The model under review builds one solid part; all positions refer to its coordinate system, in mm. A direction names the side the tool comes from. Coordinates: 2 decimals unless noted, no trailing zeros. Loops run counter-clockwise (first coordinate to the right, second up) from the corner with the lowest first, then second, coordinate; pieces in that order, holes last. Notation, with made-up numbers: M -20,-1 L 3,-1 A34 cw 3,38 Z; hole C -2.75,71.25 d5. An arc over 180 degrees is marked long. Write item = value, one per line. Start each with the question number.
Q1. For faces 1 (the face through (288.161, -6.324, 4.032)), 2 (the face through (12.161, -6.324, 4.032)), 3 (the face through (275, -7, 3)), list the 3-axis set-ups (+Z, -Z, +X, -X, +Y, -Y) from which the entire face can be reached by the end or side of a thin tool; tool diameter is ignored.
Q2. We need section B-B on x = 42.5. Give the boundary of the cut face in (y, z), and give its area (3 significant figures).
Q3. Clearance check with flat-ended pins moving along their axes: pin 1 Ø1.7 at (x, y) = (160, -1) entering from +Z; pin 2 Ø5 at (x, y) = (248, -3) entering from +Z; pin 3 Ø3 at (x, y) = (266, -4.5) entering from +Z. State where each tip first meets the part, or that it passes through.
Q4. Mouldability with a two-part tool opening along X and no side actions: class faces 4 (the face through (312, 1, 0)), 5 (the face through (152, 0, -10)), 6 (the face through (0, 1, 0)), 7 (the face through (300.76, 4.17, 2.17)) as released by +X, released by -X, zero draft, split by the parting line, or undercut.
Q5. Wall thickness on probe 1 along X at (y, z) = (6.75, 1.75); probe 2 along X at (y, z) = (1.5, -4.5); probe 3 along Y at (x, z) = (187.5, 0): over which ranges is each line inside the solid? List them lowest first.
Q6. We need section A-A on x = 159. Give the boundary of the cut face in (y, z), and give its area (3 significant figures).
from build123d import *

# Parameters (mm, degrees)
CHAMFER1_SIZE      = 0.5
SKETCH3_W          = 1.5
SKETCH3_H          = 0.3
SKETCH9_W          = 60
SKETCH9_H          = 6
CUT_EXTRUDE2_DEPTH = 3.5
FILLET4_R          = 3
FILLET5_R          = 3
FILLET6_R          = 0.2


with BuildPart() as part:
    # Sketch1 → Revolve1 (revolve)
    with BuildSketch(Plane.XY, mode=Mode.PRIVATE) as revolve1_sk:
        Polygon((0, 0), (0, 7.5), (25, 7.5), (25, 9), (26, 10), (274, 10), (275, 9), (275, 7.5), (300, 7.5), (300, 5), (312, 5), (312, 0), align=None)
    revolve(revolve1_sk.sketch.rotate(Axis((0, 0, 0), (1, 0, 0)), 90), axis=Axis((0, 0, 0), (1, 0, 0)))

    # Chamfer1
    chamfer1_edges = [part.edges().sort_by_distance(p)[0] for p in [
        (300, 0, -7.5),
        (312, 0, -5),
        (0, 0, -7.5),
    ]]
    chamfer(chamfer1_edges, length=CHAMFER1_SIZE)

    # Sketch2 → Cut-Revolve1 (revolve, cut)
    with BuildSketch(Plane.XY, mode=Mode.PRIVATE) as cut_revolve1_sk:
        Polygon((0, 0), (0, 0.5), (0.5, 0), align=None)
        Polygon((312, 0), (312, 0.5), (311.5, 0), align=None)
    revolve(cut_revolve1_sk.sketch.rotate(Axis((0, 0, 0), (1, 0, 0)), 270), axis=Axis((0, 0, 0), (1, 0, 0)), mode=Mode.SUBTRACT)

    # Sketch3 → Cut-Revolve2 (revolve, cut)
    with BuildSketch(Plane.XY, mode=Mode.PRIVATE) as cut_revolve2_sk:
        with Locations((24.25, 7.35)):
            Rectangle(SKETCH3_W, SKETCH3_H)
        with Locations((275.75, 7.35)):
            Rectangle(SKETCH3_W, SKETCH3_H)
        with Locations((300.75, 4.85)):
            Rectangle(SKETCH3_W, SKETCH3_H)
    revolve(cut_revolve2_sk.sketch.rotate(Axis((0, 0, 0), (1, 0, 0)), 90), axis=Axis((0, 0, 0), (1, 0, 0)), mode=Mode.SUBTRACT)

    # Sketch9 → Cut-Extrude2 (cut)
    with BuildSketch(Plane.XY.offset(10)):
        with Locations((150, 0)):
            Rectangle(SKETCH9_W, SKETCH9_H)
    extrude(amount=-CUT_EXTRUDE2_DEPTH, mode=Mode.SUBTRACT)

    # Fillet4
    fillet4_edges = [part.edges().sort_by_distance(p)[0] for p in [
        (120, 3, 8.019696007),
        (120, -3, 8.019696007),
    ]]
    fillet(fillet4_edges, radius=FILLET4_R - 0.0001)  # a hair under: the kernel refuses the full size

    # Fillet5
    fillet5_edges = [part.edges().sort_by_distance(p)[0] for p in [
        (180, 3, 8.019696007),
        (180, -3, 8.019696007),
    ]]
    fillet(fillet5_edges, radius=FILLET5_R - 0.0001)  # a hair under: the kernel refuses the full size

    # Fillet6
    fillet6_edges = [part.edges().sort_by_distance(p)[0] for p in [
        (150, -3, 6.5),
        (120.878650367, -2.121349633, 6.5),
        (120.878650367, 2.121349633, 6.5),
        (150, 3, 6.5),
        (179.121349633, -2.121349633, 6.5),
        (179.121349633, 2.121349633, 6.5),
    ]]
    fillet(fillet6_edges, radius=FILLET6_R)


solid = part.part
Returned:
q1.face_1 = +X
q1.face_2 = -X
q1.face_3 = none
q2.outline = C 0,0 d20
q2.area = 314 mm^2
q3.pin_1 = 6.5
q3.pin_2 = 9.99
q3.pin_3 = 9.54
q4.face_4 = released by +X
q4.face_5 = zero draft
q4.face_6 = released by -X
q4.face_7 = undercut
q5.probe_1 = 0 to 300
q5.probe_2 = 0 to 300, 301.5 to 311.76
q5.probe_3 = -10 to 10
q6.outline = M -3,6.7 L -3,9.54 A10 ccw long 3,9.54 L 3,6.7 A0.2 cw 2.8,6.5 L -2.8,6.5 A0.2 cw Z
q6.area = 294 mm^2
